Model file for the job. Use its own axes, mm. A direction names the side the tool comes from. Give positions to 0.01 mm unless a question says otherwise; leave off trailing zeros. Loops run counter-clockwise (first coordinate to the right, second up) from the corner with the lowest first, then second, coordinate; pieces in that order, holes last. Notation, with made-up numbers: M 60,85 L 73,85 A20 cw 73,96 Z; hole C 28,-13.75 d10. An arc over 180 degrees is marked long. Answer in a Markdown table with one row per item.
```python
from build123d import *
from OCP.BRepFilletAPI import BRepFilletAPI_MakeChamfer

# Parameters (mm, degrees)
BOSS_EXTRUDE1_DEPTH     = 23.2
BOSS_EXTRUDE2_START     = 23.2
BOSS_EXTRUDE2_DEPTH     = 75
CUT_EXTRUDE1_DEPTH      = 108.706127959
CUT_EXTRUDE1_DEPTH_BACK = 108.706127959
SKETCH2_W               = 2
SKETCH2_H               = 5
CUT_EXTRUDE2_DEPTH      = 108.706127959
CUT_EXTRUDE2_DEPTH_BACK = 108.706127959
BOSS_EXTRUDE3_DEPTH     = 3.2
CUT_EXTRUDE3_DEPTH      = 111.057303256
CUT_EXTRUDE3_DEPTH_BACK = 111.057303256
BOSS_EXTRUDE4_DEPTH     = 3.2
BOSS_EXTRUDE5_DEPTH     = 3.2
CUT_EXTRUDE4_DEPTH      = 3.2
CHAMFER1_SIZE           = 1.2
CHAMFER1_SIZE2          = 3.6
CHAMFER2_SIZE           = 1.2
FILLET1_R               = 0.8


with BuildPart() as part:
    # Sketch1 → Boss-Extrude1 (new body)
    with BuildSketch(Plane(origin=(0, 0, 0), x_dir=(1, 0, 0), z_dir=(0, 1, 0))):
        Polygon((-22.25475327, 13.6), (22.25475327, 13.6), (42.1, 10.359959718), (42.1, -10.359959718), (22.25475327, -13.6), (-22.25475327, -13.6), (-42.1, -10.359959718), (-42.1, 10.359959718), align=None)
    extrude(amount=BOSS_EXTRUDE1_DEPTH)

    # Sketch1<3> → Boss-Extrude2 (add)
    with BuildSketch(Plane(origin=(0, 0, 0), x_dir=(1, 0, 0), z_dir=(0, 1, 0)).offset(BOSS_EXTRUDE2_START)):
        Polygon((40.5, -9), (28.25, -11), (28.25, -8.9), (11, -8.9), (11, -12), (-11, -12), (-11, -8.9), (-28.25, -8.9), (-28.25, -11), (-40.5, -9), (-40.5, 9), (-28.25, 11), (-28.25, 8.9), (-11, 8.9), (-11, 12), (11, 12), (11, 8.9), (28.25, 8.9), (28.25, 11), (40.5, 9), align=None)
        Polygon((-38.9, -7.640040282), (-29.85, -9.117591303), (-29.85, -7.3), (-9.4, -7.3), (-9.4, -10.4), (9.4, -10.4), (9.4, -7.3), (29.85, -7.3), (29.85, -9.117591303), (38.9, -7.640040282), (38.9, 7.640040282), (29.85, 9.117591303), (29.85, 7.3), (9.4, 7.3), (9.4, 10.4), (-9.4, 10.4), (-9.4, 7.3), (-29.85, 7.3), (-29.85, 9.117591303), (-38.9, 7.640040282), align=None, mode=Mode.SUBTRACT)
    extrude(amount=BOSS_EXTRUDE2_DEPTH)

    # Sketch2 → Cut-Extrude1 (cut, two sides: drawn at the far end of the back side and taken through both)
    with BuildSketch(Plane.XY.offset(-CUT_EXTRUDE1_DEPTH_BACK)):
        with Locations((-39.5, 44.7)):
            Rectangle(SKETCH2_W, SKETCH2_H)
        with Locations((39.5, 44.7)):
            Rectangle(SKETCH2_W, SKETCH2_H)
    extrude(amount=CUT_EXTRUDE1_DEPTH + CUT_EXTRUDE1_DEPTH_BACK, mode=Mode.SUBTRACT)

    # Sketch3 → Cut-Extrude2 (cut, two sides: drawn at the far end of the back side and taken through both)
    with BuildSketch(Plane.XY.offset(-CUT_EXTRUDE2_DEPTH_BACK)):
        Polygon((-28.25, 93.2), (-19.625, 23.2), (19.625, 23.2), (28.25, 93.2), (28.25, 98.2), (-28.25, 98.2), align=None)
    extrude(amount=CUT_EXTRUDE2_DEPTH + CUT_EXTRUDE2_DEPTH_BACK, mode=Mode.SUBTRACT)

    # Sketch4 → Boss-Extrude3 (add)
    with BuildSketch(Plane(origin=(0, 0, 0), x_dir=(1, 0, 0), z_dir=(0, 1, 0))):
        Polygon((23.292779429, 26.4), (42.1, 23.329433376), (42.1, -23.329433376), (23.292779429, -26.4), (-23.292779429, -26.4), (-42.1, -23.329433376), (-42.1, 23.329433376), (-23.292779429, 26.4), align=None)
    extrude(amount=BOSS_EXTRUDE3_DEPTH)

    # Sketch1<4> → Cut-Extrude3 (cut, two sides: drawn at the far end of the back side and taken through both)
    with BuildSketch(Plane(origin=(0, 0, 0), x_dir=(1, 0, 0), z_dir=(0, 1, 0)).offset(-CUT_EXTRUDE3_DEPTH_BACK)):
        Polygon((-31.45, -5.7), (-7.8, -5.7), (-7.8, -8.8), (7.8, -8.8), (7.8, -5.7), (31.45, -5.7), (31.45, -7.235182606), (37.3, -6.280080565), (37.3, 6.280080565), (31.45, 7.235182606), (31.45, 5.7), (7.8, 5.7), (7.8, 8.8), (-7.8, 8.8), (-7.8, 5.7), (-31.45, 5.7), (-31.45, 7.235182606), (-37.3, 6.280080565), (-37.3, -6.280080565), (-31.45, -7.235182606), align=None)
    extrude(amount=CUT_EXTRUDE3_DEPTH + CUT_EXTRUDE3_DEPTH_BACK, mode=Mode.SUBTRACT)

    # Sketch5 → Boss-Extrude4 (add)
    with BuildSketch(Plane(origin=(0, 0, 0), x_dir=(1, 0, 0), z_dir=(0, 1, 0))):
        Polygon((23.292779429, 26.4), (42.1, 23.329433376), (42.1, 51.700157004), (25.563461651, 54.4), (-25.563461651, 54.4), (-42.1, 51.700157004), (-42.1, 23.329433376), (-23.292779429, 26.4), align=None)
        Polygon((-42.1, -23.329433376), (-42.1, -51.700157004), (-25.563461651, -54.4), (25.563461651, -54.4), (42.1, -51.700157004), (42.1, -23.329433376), (23.292779429, -26.4), (-23.292779429, -26.4), align=None)
    extrude(amount=BOSS_EXTRUDE4_DEPTH)

    # Sketch6 → Boss-Extrude5 (add)
    with BuildSketch(Plane(origin=(0, 0, 0), x_dir=(1, 0, 0), z_dir=(0, 1, 0))):
        Polygon((25.563461651, 54.4), (42.1, 51.700157004), (42.1, 48.100157004), (-42.1, 48.100157004), (-42.1, 51.700157004), (-25.563461651, 54.4), align=None)
        Polygon((42.1, -48.100157004), (42.1, -51.700157004), (25.563461651, -54.4), (-25.563461651, -54.4), (-42.1, -51.700157004), (-42.1, -48.100157004), align=None)
    extrude(amount=BOSS_EXTRUDE5_DEPTH)

    # Sketch7 → Cut-Extrude4 (cut)
    with BuildSketch(Plane(origin=(0, 0, 0), x_dir=(0, 0, -1), z_dir=(0, 1, 0))):
        with BuildLine():
            Line((28, -5), (28, 5))
            ThreePointArc((28, 5), (25, 8), (22, 5))
            Line((22, 5), (22, -5))
            ThreePointArc((22, -5), (25, -8), (28, -5))
        make_face()
        with BuildLine():
            Line((-28, -5), (-28, 5))
            ThreePointArc((-28, 5), (-25, 8), (-22, 5))
            Line((-22, 5), (-22, -5))
            ThreePointArc((-22, -5), (-25, -8), (-28, -5))
        make_face()
    extrude(amount=CUT_EXTRUDE4_DEPTH, mode=Mode.SUBTRACT)

    # Chamfer1: one chamfer whose edges measure the first distance from different faces: ONE call of the kernel's chamfer builder (chamfer() names one face for all edges)
    chamfer1_edges_1 = [part.edges().sort_by_distance(p)[0] for p in [
        (-33.831730825, 3.2, 53.050078502),
    ]]
    chamfer1_side_1 = [part.faces().sort_by_distance(p)[0] for p in [
        (-33.831730825, 1.6, 53.050078502),
    ]]
    chamfer1_edges_2 = [part.edges().sort_by_distance(p)[0] for p in [
        (0, 3.2, 54.4),
    ]]
    chamfer1_side_2 = [part.faces().sort_by_distance(p)[0] for p in [
        (0, 1.6, 54.4),
    ]]
    chamfer1_edges_3 = [part.edges().sort_by_distance(p)[0] for p in [
        (33.831730825, 3.2, 53.050078502),
    ]]
    chamfer1_side_3 = [part.faces().sort_by_distance(p)[0] for p in [
        (33.831730825, 1.6, 53.050078502),
    ]]
    chamfer1_edges_4 = [part.edges().sort_by_distance(p)[0] for p in [
        (33.831730825, 3.2, -53.050078502),
    ]]
    chamfer1_side_4 = [part.faces().sort_by_distance(p)[0] for p in [
        (33.831730825, 1.6, -53.050078502),
    ]]
    chamfer1_edges_5 = [part.edges().sort_by_distance(p)[0] for p in [
        (0, 3.2, -54.4),
    ]]
    chamfer1_side_5 = [part.faces().sort_by_distance(p)[0] for p in [
        (0, 1.6, -54.4),
    ]]
    chamfer1_edges_6 = [part.edges().sort_by_distance(p)[0] for p in [
        (-33.831730825, 3.2, -53.050078502),
    ]]
    chamfer1_side_6 = [part.faces().sort_by_distance(p)[0] for p in [
        (-33.831730825, 1.6, -53.050078502),
    ]]
    chamfer1 = BRepFilletAPI_MakeChamfer(part.part.solid().wrapped)
    for e in chamfer1_edges_1:
        chamfer1.Add(CHAMFER1_SIZE, CHAMFER1_SIZE2, e.wrapped, chamfer1_side_1[0].wrapped)  # the first distance lies on this face
    for e in chamfer1_edges_2:
        chamfer1.Add(CHAMFER1_SIZE, CHAMFER1_SIZE2, e.wrapped, chamfer1_side_2[0].wrapped)  # the first distance lies on this face
    for e in chamfer1_edges_3:
        chamfer1.Add(CHAMFER1_SIZE, CHAMFER1_SIZE2, e.wrapped, chamfer1_side_3[0].wrapped)  # the first distance lies on this face
    for e in chamfer1_edges_4:
        chamfer1.Add(CHAMFER1_SIZE, CHAMFER1_SIZE2, e.wrapped, chamfer1_side_4[0].wrapped)  # the first distance lies on this face
    for e in chamfer1_edges_5:
        chamfer1.Add(CHAMFER1_SIZE, CHAMFER1_SIZE2, e.wrapped, chamfer1_side_5[0].wrapped)  # the first distance lies on this face
    for e in chamfer1_edges_6:
        chamfer1.Add(CHAMFER1_SIZE, CHAMFER1_SIZE2, e.wrapped, chamfer1_side_6[0].wrapped)  # the first distance lies on this face
    add(Compound.cast(chamfer1.Shape()), mode=Mode.REPLACE)

    # Chamfer2
    chamfer2_edges = [part.edges().sort_by_distance(p)[0] for p in [
        (-42.1, 0, 0),
        (-7.8, 23.2, 7.25),
        (7.8, 23.2, 7.25),
        (7.8, 23.2, -7.25),
        (-7.8, 23.2, -7.25),
        (-7.8, 0, -7.25),
        (7.8, 0, -7.25),
        (7.8, 0, 7.25),
        (-7.8, 0, 7.25),
        (40.5, 98.2, 0),
        (28.25, 98.2, -9.15),
        (-28.25, 98.2, 9.15),
        (0, 0, 54.4),
        (33.831730825, 0, 53.050078502),
        (-33.831730825, 0, 53.050078502),
        (33.831730825, 0, -53.050078502),
        (0, 0, -54.4),
        (-33.831730825, 0, -53.050078502),
        (28.25, 98.2, 9.15),
        (-28.25, 98.2, -9.15),
        (-40.5, 98.2, 0),
        (42.1, 0, 0),
    ]]
    chamfer(chamfer2_edges, length=CHAMFER2_SIZE)

    # Fillet1
    fillet1_edges = [part.edges().sort_by_distance(p)[0] for p in [
        (-42.1, 13.2, 10.359959718),
        (42.1, 13.2, 10.359959718),
        (42.1, 13.2, -10.359959718),
        (-42.1, 13.2, -10.359959718),
        (-42.1, 1.6, 51.700157004),
        (-42.1, 1.6, -51.700157004),
        (42.1, 1.6, -51.700157004),
        (42.1, 1.6, 51.700157004),
    ]]
    fillet(fillet1_edges, radius=FILLET1_R)


solid = part.part
```
(1) Wall check: L1, parallel to Z at x = -13, y = 15; L2, parallel to X at y = 91, z = -3; L3, parallel to Y at x = 5, z = 31.5. Give the ranges that are in metal, low to high.
Established:
| item | result |
|---|---|
| L1 | z = -13.6 to -5.7, 5.7 to 13.6 |
| L2 | x = -40.5 to -38.9, 38.9 to 40.5 |
| L3 | y = 0 to 3.2 |
(2) Flat gauge pins, fed straight in: P1, Ø8, axis at x = -0.5, z = 35.5, coming from the +Y side; P2, Ø7, axis at x = 17, y = 12.5, coming from the +Z side; P3, Ø4, axis at x = 33, y = 29.5, coming from the -Z side; P4, Ø3, axis at x = 23, y = 73, coming from the -Z side. Where does each tip first touch, or does it go through?
Established:
| item | result |
|---|---|
| P1 | stops at y = 3.2 |
| P2 | stops at z = 13.6 |
| P3 | stops at z = -10.55 |
| P4 | passes through |
(3) Saw through at C-C, the plane x = 0.5. Give the cut face in (y, z).
Established:
| item | result |
|---|---|
| outline | M 0,-53.2 L 1.2,-54.4 L 2,-54.4 L 3.2,-50.8 L 3.2,-28 L 0,-28 Z; M 0,-22 L 3.2,-22 L 3.2,-13.6 L 23.2,-13.6 L 23.2,-8.8 L 0,-8.8 Z; M 0,8.8 L 23.2,8.8 L 23.2,13.6 L 3.2,13.6 L 3.2,22 L 0,22 Z; M 0,28 L 3.2,28 L 3.2,50.8 L 2,54.4 L 1.2,54.4 L 0,53.2 Z |
(4) Saw through at D-D, the plane z = 25. Give the cut face in (x, y).
Established:
| item | result |
|---|---|
| outline | M -42.1,1.2 L -40.9,0 L -8,0 L -8,3.2 L -42.1,3.2 Z; M 8,0 L 40.9,0 L 42.1,1.2 L 42.1,3.2 L 8,3.2 Z |
(5) Mould opens along Z. For faces 4 (the flat face through (0, 11, 8.8)), 5 (the flat face through (0, 13, 13.6)), 6 (the flat face through (39.1, 98.2, -0.1)) say: pulls with the +Z half, pulls with the -Z half, needs draft (parallel to the pull), parting line crosses it, or undercut.
Established:
| item | result |
|---|---|
| face 4 | undercut |
| face 5 | pulls with the +Z half |
| face 6 | needs draft |
(6) Saw through at A-A, the plane x = -10.5. Give the cut face in (y, z).
Established:
| item | result |
|---|---|
| outline | M 0,-53.2 L 1.2,-54.4 L 2,-54.4 L 3.2,-50.8 L 3.2,-13.6 L 23.2,-13.6 L 23.2,-5.7 L 0,-5.7 Z; M 0,5.7 L 23.2,5.7 L 23.2,13.6 L 3.2,13.6 L 3.2,50.8 L 2,54.4 L 1.2,54.4 L 0,53.2 Z |
(7) Which spindle directions (+Z, -Z, +X, -X, +Y, -Y) get a long thin tool onto all of the face, cutting with end or side? Do faces 1 (the flat face through (34.289, 60.175, -10.014)), 2 (the flat face through (34.42, 11.44, -6.75)), 3 (the flat face through (26, 52, -7.3)). Say none if no direction does.
Established:
| item | result |
|---|---|
| face 1 | -Z, +X, +Y |
| face 2 | +Y, -Y |
| face 3 | +Y |
